Source: CAD feature listing. Evaluate the final solid. Frame: model axes, mm. A direction names the side the tool comes from. Give positions to 0.01 mm unless a question says otherwise; leave off trailing zeros. Loops run counter-clockwise (first coordinate to the right, second up) from the corner with the lowest first, then second, coordinate; pieces in that order, holes last. Notation, with made-up numbers: M 20.5,63.5 L 70.5,63.5 A14 cw 70.5,70.5 Z; hole C 19,-17 d5. An arc over 180 degrees is marked long. Answer in a Markdown table with one row per item.
```python
from build123d import *

# Parameters (mm, degrees)
SKETCH1_R           = 41
SKETCH1_R_2         = 15
BOSS_EXTRUDE1_DEPTH = 14.5
SKETCH3_W           = 12
SKETCH3_H           = 9
HOLE1_D             = 4
HOLE1_CBORE_D       = 7
HOLE1_CBORE_DEPTH   = 2.8
CIRPATTERN1_COUNT   = 8


with BuildPart() as part:
    # Sketch1 → Boss-Extrude1 (new body, symmetric)
    with BuildSketch(Plane(origin=(0, 0, 0), x_dir=(1, 0, 0), z_dir=(0, 1, 0))):
        Circle(SKETCH1_R)
        Circle(SKETCH1_R_2, mode=Mode.SUBTRACT)
    extrude(amount=BOSS_EXTRUDE1_DEPTH, both=True)

    # Sketch3 → Cut-Revolve1 (revolve, cut)
    with BuildSketch(Plane(origin=(0, 0, 0), x_dir=(0, 0, -1), z_dir=(1, 0, 0))):
        with Locations((35, 0)):
            Rectangle(SKETCH3_W, SKETCH3_H)
    revolve(axis=Axis((0, 14.5, 0), (0, -1, 0)), mode=Mode.SUBTRACT)

    # Hole1 (through all)
    with Locations(Plane(origin=(0, 14.5, -21.25), x_dir=(0, 0, 1), z_dir=(0, 1, 0))):
        with Locations((0, 0)):
            hole1 = CounterBoreHole(HOLE1_D / 2, HOLE1_CBORE_D / 2, HOLE1_CBORE_DEPTH)

    # CirPattern1: Hole1 ×8 about axis
    cirpattern1_axis = Axis((0, 0, 0), (0, 1, 0))
    for i in range(1, CIRPATTERN1_COUNT):
        add(hole1.rotate(cirpattern1_axis, i * 360 / CIRPATTERN1_COUNT), mode=Mode.SUBTRACT)


solid = part.part
```
1) Material intervals for L1, parallel to Y at x = 1, z = 36; L2, parallel to Z at x = 16, y = -2.75; L3, parallel to Z at x = 0.5, y = 10, sorted ascending.
Reply:
| item | result |
|---|---|
| L1 | y = -14.5 to -4.5, 4.5 to 14.5 |
| L2 | z = -24.19 to -16.77, -13.28 to 13.28, 16.77 to 24.19 |
| L3 | z = -41 to -23.19, -19.31 to -14.99, 14.99 to 19.31, 23.19 to 41 |
2) Section D-D, the plane x = -21.25. Return loops of the section in (y, z).
Reply:
| item | result |
|---|---|
| outline | M -14.5,-35.06 L -4.5,-35.06 L -4.5,-19.73 L 4.5,-19.73 L 4.5,-35.06 L 14.5,-35.06 L 14.5,-3.5 L 11.7,-3.5 L 11.7,-2 L -14.5,-2 Z; M -14.5,2 L 11.7,2 L 11.7,3.5 L 14.5,3.5 L 14.5,35.06 L 4.5,35.06 L 4.5,19.73 L -4.5,19.73 L -4.5,35.06 L -14.5,35.06 Z |
3) Set-up query: faces 5 (the cylindrical face through (-14.594, -1.583, -16.979)), 6 (the cylindrical face through (-17.6, 13.1, 17.4)). Return all of +Z, -Z, +X, -X, +Y, -Y with unobstructed straight access to the full face (end or side cutting, diameter ignored); none if empty.
Reply:
| item | result |
|---|---|
| face 5 | +Y, -Y |
| face 6 | +Y |
4) Section A-A, the plane z = 0. Count the separate pieces of the cut face and the enclosed holes in it, then the cut area to 3 significant figures.
Reply:
| item | result |
|---|---|
| separate pieces | 4 |
| enclosed holes | 0 |
| area | 1,040 mm² |
5) Pull-direction query (X, two-part tool) for faces 1 (the flat face through (18, -14.5, -1)), 2 (the cylindrical face through (-1.05, 13.12, 17.91)), 3 (the cylindrical face through (37.874, -9.43, 15.703)), 4 (the cylindrical face through (16.8, -1.58, -15.95)); classes: released by +X, released by -X, zero draft, split by the parting line, or undercut.
Reply:
| item | result |
|---|---|
| face 1 | zero draft |
| face 2 | undercut |
| face 3 | split by the parting line |
| face 4 | undercut |
6) Section C-C, the plane z = -20.5. Return loops of the section in (x, y), then the cut area to 3 significant figures.
Reply:
| item | result |
|---|---|
| outline | M -35.51,-14.5 L -1.85,-14.5 L -1.85,11.7 L -3.42,11.7 L -3.42,14.5 L -35.51,14.5 L -35.51,4.5 L -20.51,4.5 L -20.51,-4.5 L -35.51,-4.5 Z; M 1.85,-14.5 L 35.51,-14.5 L 35.51,-4.5 L 20.51,-4.5 L 20.51,4.5 L 35.51,4.5 L 35.51,14.5 L 3.42,14.5 L 3.42,11.7 L 1.85,11.7 Z |
| area | 1,670 mm² |
7) Pin query (flat end, axial travel): pin 1 Ø4 at (y, z) = (-11, -26.5) entering from -X; pin 2 Ø12 at (y, z) = (-5.5, -16.5) entering from +X; pin 3 Ø4.5 at (x, z) = (21.25, 0) entering from +Y. Return the tip coordinate at first contact, or that it passes through.
Reply:
| item | result |
|---|---|
| pin 1 | stops at x = -32.87 |
| pin 2 | stops at x = 39.63 |
| pin 3 | stops at y = 11.7 |
